from build123d import *

# Parameters (mm, degrees)
SKETCH1_R           = 1
BOSS_EXTRUDE1_DEPTH = 1.5


with BuildPart() as part:
    # Sketch1 → Boss-Extrude1 (new, symmetric)
    with BuildSketch(Plane.XY):
        with BuildLine():
            Line((30.5, 37.5), (30.5, 25.5))
            Line((30.5, 25.5), (53, 25.5))
            Line((53, 25.5), (53, 37.5))
            Line((53, 37.5), (60, 37.5))
            ThreePointArc((60, 37.5), (63.535533906, 36.035533906), (65, 32.5))
            Line((65, 32.5), (65, 28.283390528))
            ThreePointArc((65, 28.283390528), (64.524852545, 26.15601904), (63.189716221, 24.432973612))
            Line((63.189716221, 24.432973612), (58.820567558, 20.813535857))
            ThreePointArc((58.820567558, 20.813535857), (56.15029491, 17.367445), (55.2, 13.112702024))
            Line((55.2, 13.112702024), (55.2, -13.112702024))
            ThreePointArc((55.2, -13.112702024), (56.15029491, -17.367445), (58.820567558, -20.813535857))
            Line((58.820567558, -20.813535857), (63.189716221, -24.432973612))
            ThreePointArc((63.189716221, -24.432973612), (64.524852545, -26.15601904), (65, -28.283390528))
            Line((65, -28.283390528), (65, -32.5))
            ThreePointArc((65, -32.5), (63.535533906, -36.035533906), (60, -37.5))
            Line((60, -37.5), (53, -37.5))
            Line((53, -37.5), (53, -25.5))
            Line((53, -25.5), (30.5, -25.5))
            Line((30.5, -25.5), (30.5, -37.5))
            Line((30.5, -37.5), (24.141964056, -37.5))
            Line((24.141964056, -37.5), (24.141964056, -35.5))
            ThreePointArc((24.141964056, -35.5), (21.213031868, -28.428932188), (14.141964056, -25.5))
            Line((14.141964056, -25.5), (-14.141964056, -25.5))
            ThreePointArc((-14.141964056, -25.5), (-21.213031868, -28.428932188), (-24.141964056, -35.5))
            Line((-24.141964056, -35.5), (-24.141964056, -37.5))
            Line((-24.141964056, -37.5), (-30.5, -37.5))
            Line((-30.5, -37.5), (-30.5, -25.5))
            Line((-30.5, -25.5), (-53, -25.5))
            Line((-53, -25.5), (-53, -37.5))
            Line((-53, -37.5), (-60, -37.5))
            ThreePointArc((-60, -37.5), (-63.535533906, -36.035533906), (-65, -32.5))
            Line((-65, -32.5), (-65, -28.283390528))
            ThreePointArc((-65, -28.283390528), (-64.524852545, -26.15601904), (-63.189716221, -24.432973612))
            Line((-63.189716221, -24.432973612), (-58.820567558, -20.813535857))
            ThreePointArc((-58.820567558, -20.813535857), (-56.15029491, -17.367445), (-55.2, -13.112702024))
            Line((-55.2, -13.112702024), (-55.2, 13.112702024))
            ThreePointArc((-55.2, 13.112702024), (-56.15029491, 17.367445), (-58.820567558, 20.813535857))
            Line((-58.820567558, 20.813535857), (-63.189716221, 24.432973612))
            ThreePointArc((-63.189716221, 24.432973612), (-64.524852545, 26.15601904), (-65, 28.283390528))
            Line((-65, 28.283390528), (-65, 32.5))
            ThreePointArc((-65, 32.5), (-63.535533906, 36.035533906), (-60, 37.5))
            Line((-60, 37.5), (-53, 37.5))
            Line((-53, 37.5), (-53, 25.5))
            Line((-53, 25.5), (-30.5, 25.5))
            Line((-30.5, 25.5), (-30.5, 37.5))
            Line((-30.5, 37.5), (-24.141964056, 37.5))
            Line((-24.141964056, 37.5), (-24.141964056, 35.5))
            ThreePointArc((-24.141964056, 35.5), (-21.213031868, 28.428932188), (-14.141964056, 25.5))
            Line((-14.141964056, 25.5), (14.141964056, 25.5))
            ThreePointArc((14.141964056, 25.5), (21.213031868, 28.428932188), (24.141964056, 35.5))
            Line((24.141964056, 35.5), (24.141964056, 37.5))
            Line((24.141964056, 37.5), (30.5, 37.5))
        make_face()
        with Locations((55.2, 31.4)):
            Circle(SKETCH1_R, mode=Mode.SUBTRACT)
        with Locations(Location((28.3, 31.4, 0), (0, 0, 180))):
            Circle(SKETCH1_R, mode=Mode.SUBTRACT)
        with Locations((-28.3, 31.4)):
            Circle(SKETCH1_R, mode=Mode.SUBTRACT)
        with Locations(Location((-28.3, -31.4, 0), (0, 0, 180))):
            Circle(SKETCH1_R, mode=Mode.SUBTRACT)
        with Locations((28.3, -31.4)):
            Circle(SKETCH1_R, mode=Mode.SUBTRACT)
        with Locations(Location((55.2, -31.4, 0), (0, 0, 180))):
            Circle(SKETCH1_R, mode=Mode.SUBTRACT)
        with Locations(Location((-55.2, 31.4, 0), (0, 0, 180))):
            Circle(SKETCH1_R, mode=Mode.SUBTRACT)
        with Locations((-55.2, -31.4)):
            Circle(SKETCH1_R, mode=Mode.SUBTRACT)
    extrude(amount=BOSS_EXTRUDE1_DEPTH, both=True)


solid = part.part
The listing builds one solid part. Answer for the finished solid, in the listing's coordinates (mm). A direction names the side the tool comes from. Give positions to 0.01 mm unless a question says otherwise; leave off trailing zeros. Write each loop counter-clockwise with the first axis right and the second up, starting at its lowest first coordinate (ties: lowest second). Pieces come first, ordered by that corner, then holes.
1) Find the intervals of material crossed by L1, parallel to Y at x = -28.3, z = -0.5; L2, parallel to X at y = -33, z = 0.65; L3, parallel to X at y = -29, z = -0.1, in increasing order.
2) Section B-B (x = -37) is taken. Write down the section's boundary in (y, z), and give its area (3 significant figures).
3) For a pull along Y with two mould halves and no side action, classify faces 5 (the face through (-27, 37.5, 0)), 6 (the face through (-53, 32, 0)), 7 (the face through (-55.2, 0, 0)) as pulls with the +Y half, pulls with the -Y half, needs draft (parallel to the pull), parting line crosses it, or undercut.
4) A tool of negligible diameter and unlimited length cuts with its end or side. For faces 1 (the face through (-64.538, -26.184, 0.021)), 2 (the face through (-42, 25.5, 0)), 3 (the face through (-30.5, -32, 0)), 4 (the face through (61.04, 22.65, 0.02)), from which of +Z, -Z, +X, -X, +Y, -Y can it reach the whole face along a straight path? Write none if from no direction.
5) Given P1, Ø1.6, axis at x = -28.3, y = -31.4, coming from the -Z side; P2, Ø1.5, axis at x = 1, z = 0.5, coming from the +Y side; P3, Ø1.5, axis at x = -43.5, z = 0.5, coming from the -Y side; P4, Ø1, axis at y = 27, z = 0.5, coming from the +X side, each flat-ended and moving along its own axis, determine where each tip first touches the part or whether it passes through.
6) Section C-C (y = 7) is taken. Write down the section's boundary in (x, z), and give its area (3 significant figures).
7) Section A-A (z = 0.8) is taken. Count the separate pieces of the cut face and the enclosed holes in it, and give its area (3 significant figures).
Response:
1. L1: y = -37.5 to -32.4, -30.4 to 30.4, 32.4 to 37.5
1. L2: x = -64.97 to -53, -30.5 to -23.82, 23.82 to 30.5, 53 to 64.97
1. L3: x = -65 to -53, -30.5 to -21.74, 21.74 to 30.5, 53 to 65
2. outline: (-25.5, -1.5) - (25.5, -1.5) - (25.5, 1.5) - (-25.5, 1.5) - close
2. area: 153 mm2
3. face 5: pulls with the +Y half
3. face 6: needs draft
3. face 7: undercut
4. face 1: +Z, -Z, -X
4. face 2: +Z, -Z, +Y
4. face 3: +Z, -Z, -Y
4. face 4: +Z, -Z, +X
5. P1: passes through
5. P2: stops at y = 25.5
5. P3: stops at y = -25.5
5. P4: stops at x = 64.94
6. outline: (-55.2, -1.5) - (55.2, -1.5) - (55.2, 1.5) - (-55.2, 1.5) - close
6. area: 331 mm2
7. separate pieces: 1
7. enclosed holes: 8
7. area: 6,700 mm2
